Check sheet for the drawn part. Datum: minimum x, y, z corner. Units: mm. A direction names the side the tool comes from. Round coordinates to 2 decimals unless told otherwise and drop trailing zeros. Write each loop counter-clockwise with the first axis right and the second up, starting at its lowest first coordinate (ties: lowest second). Pieces come first, ordered by that corner, then holes. Notation, with made-up numbers: M 73.25,15 L 109.25,15 A17 cw 109.25,37 Z; hole C -12,37 d9. An arc over 180 degrees is marked long. Use a Markdown table: item, result.
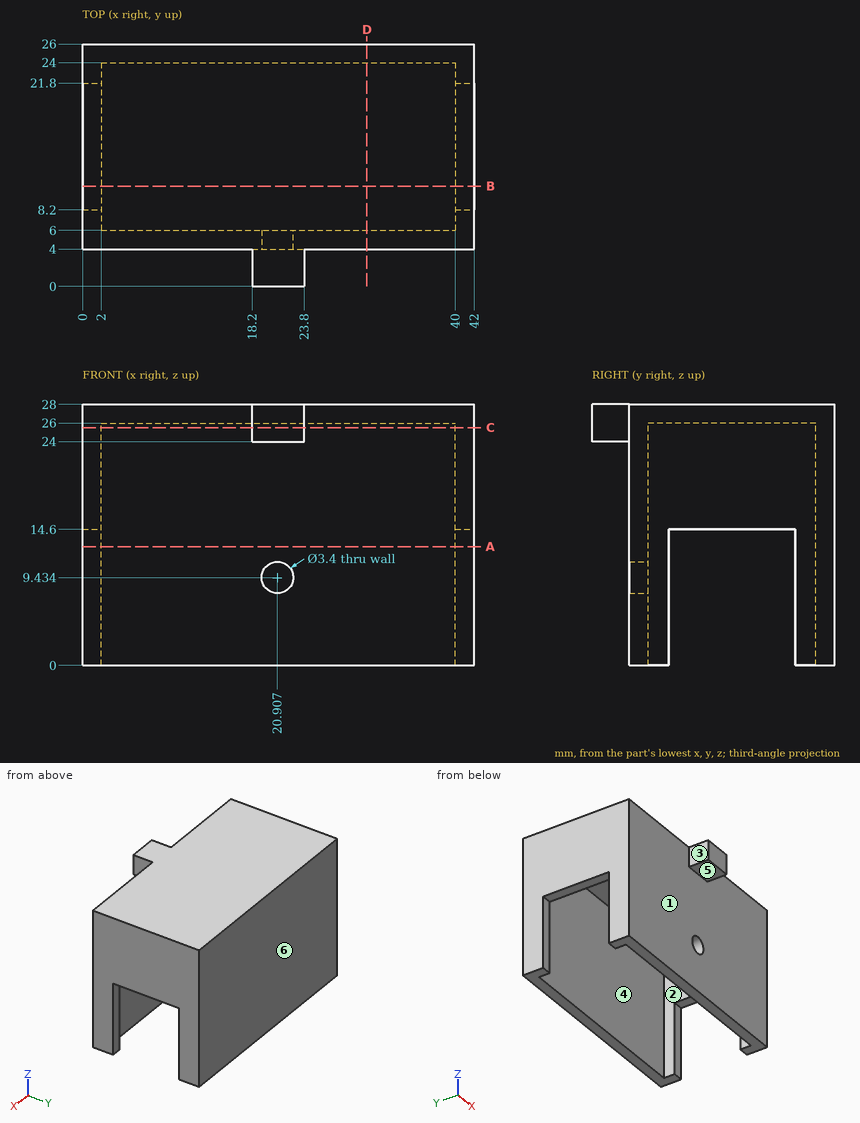
Item 1: Cross-section at A-A, the plane z = 12.75. Record the cut outline in (x, y).
Outcome:
| item | result |
|---|---|
| outline | M 0,4 L 42,4 L 42,8.2 L 40,8.2 L 40,6 L 2,6 L 2,8.2 L 0,8.2 Z; M 0,21.8 L 2,21.8 L 2,24 L 40,24 L 40,21.8 L 42,21.8 L 42,26 L 0,26 Z |
Item 2: Cross-section at C-C, the plane z = 25.5. Record the cut outline in (x, y).
Outcome:
| item | result |
|---|---|
| outline | M 0,4 L 18.2,4 L 18.2,0 L 23.8,0 L 23.8,4 L 42,4 L 42,26 L 0,26 Z; hole M 2,6 L 40,6 L 40,24 L 2,24 Z |
Item 3: Access from +Z, -Z, +X, -X, +Y, -Y to the whole of each face (thin tool, end or side, straight path). Record for the marked faces 4, 5 and 6.
Outcome:
| item | result |
|---|---|
| face 4 | -Z |
| face 5 | -Z, +X, -X, -Y |
| face 6 | +Z, -Z, +X, -X, +Y |
Item 4: Cross-section at B-B, the plane y = 10.75. Record the cut outline in (x, z), and give its area (3 significant figures).
Outcome:
| item | result |
|---|---|
| outline | M 0,14.6 L 2,14.6 L 2,26 L 40,26 L 40,14.6 L 42,14.6 L 42,28 L 0,28 Z |
| area | 130 mm2 |
Item 5: Cross-section at D-D, the plane x = 30.5. Record the cut outline in (y, z), and give its area (3 significant figures).
Outcome:
| item | result |
|---|---|
| outline | M 4,0 L 6,0 L 6,26 L 24,26 L 24,0 L 26,0 L 26,28 L 4,28 Z |
| area | 148 mm2 |
Item 6: Material ranges on line 1 along Y through (x, z) = (36.5, 2.25); line 2 along X through (y, z) = (11, 18); line 3 along Z through (x, y) = (25.5, 20.25), recorded low to high. Write a range as from..to.
Outcome:
| item | result |
|---|---|
| line 1 | y = 4..6, 24..26 |
| line 2 | x = 0..2, 40..42 |
| line 3 | z = 26..28 |
Item 7: Mould release check, pull along X, two halves, no side actions. Record for the marked faces 1, 2 and 3: +X half, -X half, draft (parallel to the pull), parting line (faces both ways), or undercut.
Outcome:
| item | result |
|---|---|
| face 1 | draft |
| face 2 | undercut |
| face 3 | -X half |
Item 8: Go/stop test with flat-tipped pins: pin 1 (1.2 mm diameter, centred on y = 2, z = 26.5, fed in from -X); pin 2 (10 mm diameter, centred on x = 12, y = 17.5, fed in from -Z); pin 3 (14 mm diameter, centred on x = 24, z = 14.5, fed in from -Y). Record where each tip stops, or that it passes through.
Outcome:
| item | result |
|---|---|
| pin 1 | stops at x = 18.2 |
| pin 2 | stops at z = 26 |
| pin 3 | stops at y = 4 |
